Read the model definition and answer for the solid it produces. Units are mm, in the model's axes. A direction names the side the tool comes from. Coordinates: 2 decimals unless noted, no trailing zeros. Loops run counter-clockwise (first coordinate to the right, second up) from the corner with the lowest first, then second, coordinate; pieces in that order, holes last.
Q1. Section B-B (y = -593) is taken. Give the vertices of the cut face in (x, z).
Q2. Straight lines are drawn through the part: line 1 (X direction, y = -415.5, z = 262); line 2 (Z direction, x = 215, y = -611); line 3 (Z direction, x = 115, y = 417.5). For each, find the intervals that lie inside material, in ascending order.
Q3. Section C-C (x = 269) is taken. Give the vertices of the cut face in (y, z).
Q4. Flat-ended cylindrical pins translate along their axes: P1, Ø3, axis at x = -63, y = 88, coming from the +Z side; P2, Ø3, axis at x = -412, y = -305, coming from the -Z side; P3, Ø1.5, axis at y = -551, z = 267, coming from the -X side; P4, Ø21, axis at y = 686, z = 754.5, coming from the +X side. Find the tip coordinate at first contact, or state that the pin passes through.
Q5. The mould has two halves that part along X. Classify faces 4 (the face through (302, -385, 330.2)), 5 (the face through (533.4, -10, 172)), 6 (the face through (-7, 10, 0)): pulls with the +X half, pulls with the -X half, needs draft (parallel to the pull), parting line crosses it, or undercut.
Q6. Which of the six approach directions +Z, -Z, +X, -X, +Y, -Y give full straight-line access (tool end or side, diameter ignored) to faces 1 (the face through (-239, 679.45, 620)), 2 (the face through (302, -385, 19.05)), 3 (the face through (77, -698.5, 96))?
Q7. Section D-D (y = 585.5) is taken. Give the vertices of the cut face in (x, z).
Q8. Section A-A (z = 227.5) is taken. Give the vertices of the cut face in (x, y).
from build123d import *

# Parameters (mm, degrees)
F0_W     = 1066.8
F0_H     = 1397
F1_DEPTH = 19.05
F2_W     = 457.2
F2_H     = 1397
F3_DEPTH = 330.2
F4_W     = 597.298336
F4_H     = 19.05
F5_DEPTH = 1219.2
F6_W     = 419.1
F6_H     = 311.15
F7_DEPTH = 635


with BuildPart() as f1:
    # F0 (on Top) → F1 (new body)
    with BuildSketch(Plane.XY):
        Rectangle(F0_W, F0_H)
    extrude(amount=F1_DEPTH)

    # F2 (on face) → F3 (join)
    with BuildSketch(Plane.XY.offset(19.05)):
        with Locations((304.8, 0)):
            Rectangle(F2_W, F2_H)
    extrude(amount=F3_DEPTH)

    # F4 (on face) → F5 (join)
    with BuildSketch(Plane.XY.offset(19.05)):
        with Locations((-234.750832, 688.975)):
            Rectangle(F4_W, F4_H)
    extrude(amount=F5_DEPTH)

    # F6 (on face) → F7 (cut)
    with BuildSketch(Plane.XZ.offset(698.5)):
        with Locations((304.8, 174.625)):
            Rectangle(F6_W, F6_H)
    extrude(amount=-F7_DEPTH, mode=Mode.SUBTRACT)


solid = f1.part
Numbers:
1. outline: (-533.4, 0) - (533.4, 0) - (533.4, 349.25) - (76.2, 349.25) - (76.2, 19.05) - (-533.4, 19.05) - close; hole (95.25, 19.05) - (514.35, 19.05) - (514.35, 330.2) - (95.25, 330.2) - close
2. line 1: x = 76.2 to 95.25, 514.35 to 533.4
2. line 2: z = 0 to 19.05, 330.2 to 349.25
2. line 3: z = 0 to 349.25
3. outline: (-698.5, 0) - (698.5, 0) - (698.5, 349.25) - (-698.5, 349.25) - (-698.5, 330.2) - (-63.5, 330.2) - (-63.5, 19.05) - (-698.5, 19.05) - close
4. P1: stops at z = 19.05
4. P2: stops at z = 0
4. P3: stops at x = 76.2
4. P4: stops at x = 63.9
5. face 4: undercut
5. face 5: pulls with the +X half
5. face 6: needs draft
6. face 1: +Z, -X, -Y
6. face 2: -Y
6. face 3: +Z, -Z, +X, -X, -Y
7. outline: (-533.4, 0) - (533.4, 0) - (533.4, 349.25) - (76.2, 349.25) - (76.2, 19.05) - (-533.4, 19.05) - close
8. outline: (-533.4, 679.45) - (63.9, 679.45) - (63.9, 698.5) - (-533.4, 698.5) - close; (76.2, -698.5) - (95.25, -698.5) - (95.25, -63.5) - (514.35, -63.5) - (514.35, -698.5) - (533.4, -698.5) - (533.4, 698.5) - (76.2, 698.5) - close
